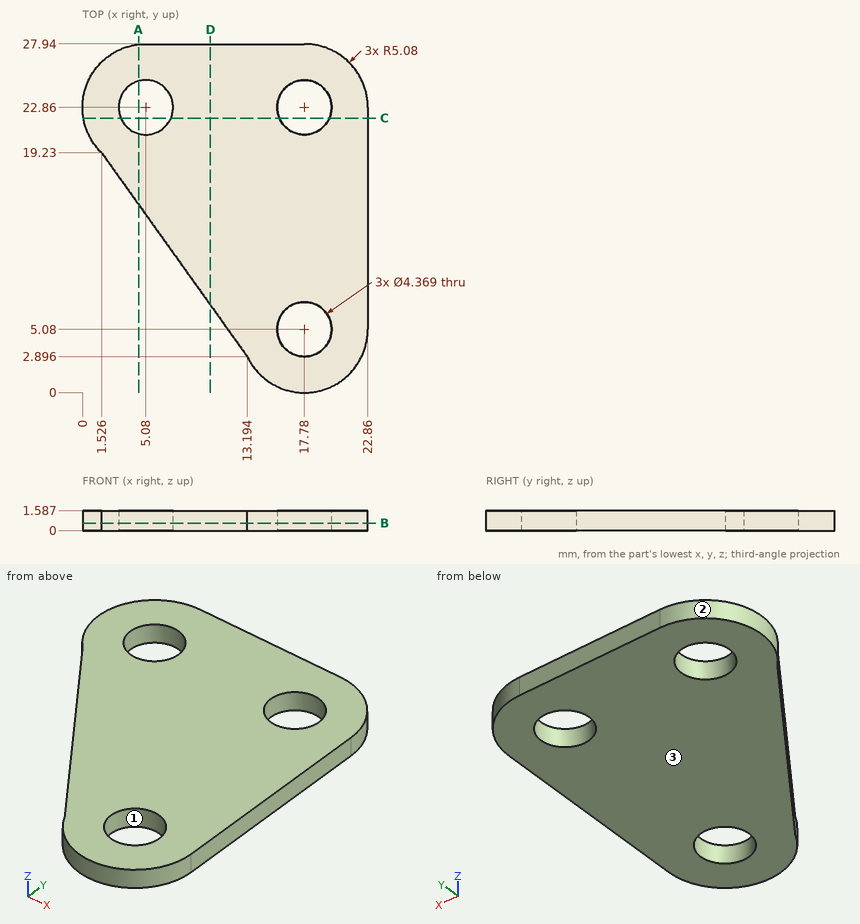
Can you work these out from the drawing? Everything is in mm from the part's minimum corner. Give positions to 0.01 mm unless a question says otherwise; leave off trailing zeros. Loops run counter-clockwise (first coordinate to the right, second up) from the corner with the lowest first, then second, coordinate; pieces in that order, holes last. Notation, with made-up numbers: M -21,-25.5 L -10,-25.5 A22 cw -10,-3.5 Z; hole C 77,55.5 d2. An arc over 180 degrees is marked long. Put each result on its own line as item: value. Start each with the question number.
(1) If we mould it in two halves opening along Y, with no side actions, what happens to the marked faces 1, 2 and 3? For each: +Y half, -Y half, draft (parallel to the pull), parting line (faces both ways), or undercut.
(2) I want a section at D-D on x = 10.25. Please give me the cut outline in (y, z).
(3) I need wall thicknesses on line 1 along Y through (x, z) = (17.78, 1.25) (1 decimal); line 2 along Y through (x, z) = (5.08, 1.15) (1 decimal); line 3 along Y through (x, z) = (17.25, 0.7). Which ranges of each line are inside material? Lowest first, please. Write a range as [from, to].
(4) I want a section at C-C on y = 22. Please give me the cut outline in (x, z).
(5) I want a section at B-B on z = 0.6. Please give me the cut outline in (x, y) (1 decimal).
(6) I want a section at A-A on x = 4.5. Please give me the cut outline in (y, z) (1 decimal).
Answer block:
1. face 1: undercut
1. face 2: parting line
1. face 3: draft
2. outline: M 7.02,0 L 27.94,0 L 27.94,1.59 L 7.02,1.59 Z
3. line 1: [0, 2.9], [7.3, 20.7], [25, 27.9]
3. line 2: [14.3, 20.7], [25, 27.9]
3. line 3: [0.03, 2.96], [7.2, 20.74], [24.98, 27.94]
4. outline: M 0.07,0 L 3.07,0 L 3.07,1.59 L 0.07,1.59 Z; M 7.09,0 L 15.77,0 L 15.77,1.59 L 7.09,1.59 Z; M 19.79,0 L 22.86,0 L 22.86,1.59 L 19.79,1.59 Z
5. outline: M 1.5,19.2 L 13.2,2.9 A5.1 ccw 22.9,5.1 L 22.9,22.9 A5.1 ccw 17.8,27.9 L 5.1,27.9 A5.1 ccw Z; hole C 5.1,22.9 d4.4; hole C 17.8,5.1 d4.4; hole C 17.8,22.9 d4.4
6. outline: M 15.1,0 L 20.8,0 L 20.8,1.6 L 15.1,1.6 Z; M 25,0 L 27.9,0 L 27.9,1.6 L 25,1.6 Z
